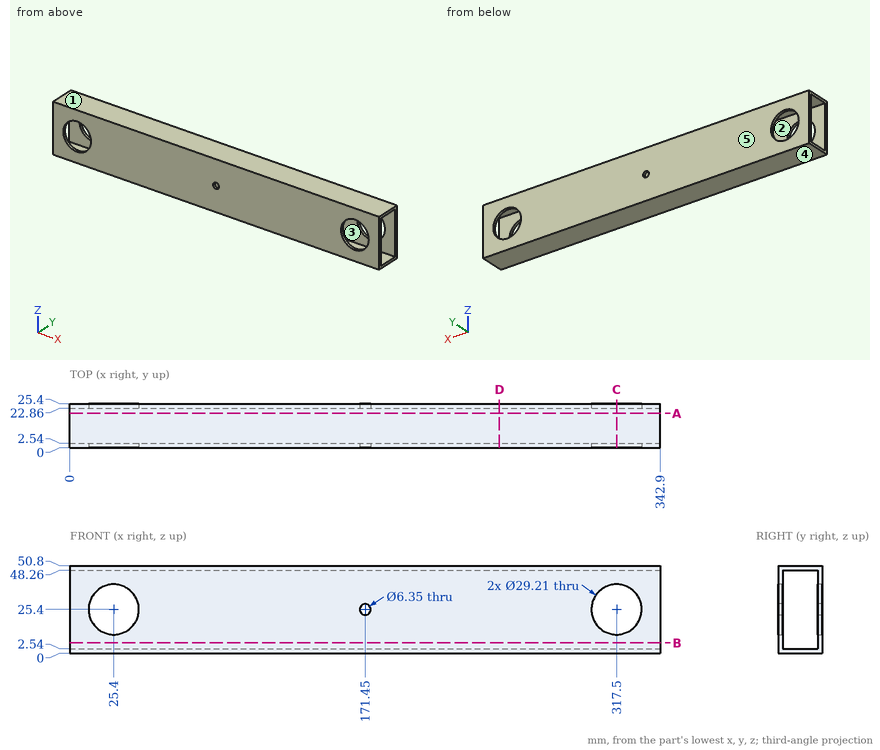
Job drawing, mm, ordinate dimensions from the low corner. One solid piece. A direction names the side the tool comes from. Coordinates: 2 decimals unless noted, no trailing zeros. Loops run counter-clockwise (first coordinate to the right, second up) from the corner with the lowest first, then second, coordinate; pieces in that order, holes last. Notation, with made-up numbers: (-36, -5.75) - (-17, -5.75) arc R19 cw to (-17, 11.25) - close; hole circle Ø3 at (29, 80). An arc over 180 degrees is marked (long way). Answer as a JSON object with one key per item and string values. Group by question number.
(1) Flat gauge pins, fed straight in: pin 1 (1.5 mm diameter, centred on x = 43.5, y = 17, fed in from -Z); pin 2 (10 mm diameter, centred on y = 17.5, z = 20.5, fed in from +X). Where does each tip first touch, or does it go through?
(2) Cut at D-D (x = 249.5). Give the cut face in (y, z).
(3) Two-plate mould, pull along Z, no slides. Class the marked faces 3, 4 and 5: released by +Z, released by -Z, zero draft, split by the parting line, or undercut.
(4) Tool access for the marked faces 1 and 2: list every direction of +Z, -Z, +X, -X, +Y, -Y with a clear straight run to the whole face (end or side of a thin tool).
(5) Cut at C-C (x = 317.5). Give the cut face in (y, z) (3 decimals), then the cut area to 3 significant figures.
(6) Probe line 1 along X through (y, z) = (1.85, 25.4) (3 decimals); line 2 along Z through (x, y) = (82.5, 22.25); line 3 along Y through (x, z) = (36.5, 35). List the from-to ranges inside material, lowest first.
(7) Cut at A-A (y = 20). Give the cut face in (x, z), then the cut area to 3 significant figures.
(8) Cut at B-B (z = 6). Give the cut face in (x, y), then the cut area to 3 significant figures.
Geometry says:
{
 "1": {"pin 1": "stops at z = 0", "pin 2": "passes through"},
 "2": {"outline": "(0, 0) - (25.4, 0) - (25.4, 50.8) - (0, 50.8) - close; hole (2.54, 2.54) - (22.86, 2.54) - (22.86, 48.26) - (2.54, 48.26) - close"},
 "3": {"face 3": "undercut", "face 4": "released by -Z", "face 5": "zero draft"},
 "4": {"face 1": "+Z, +X, -X, +Y, -Y", "face 2": "+X, -X"},
 "5": {"outline": "(0, 0) - (25.4, 0) - (25.4, 10.795) - (22.86, 10.795) - (22.86, 2.54) - (2.54, 2.54) - (2.54, 10.795) - (0, 10.795) - close; (0, 40.005) - (2.54, 40.005) - (2.54, 48.26) - (22.86, 48.26) - (22.86, 40.005) - (25.4, 40.005) - (25.4, 50.8) - (0, 50.8) - close", "area": "213 mm^2"},
 "6": {"line 1": "x = 0 to 10.795, 40.005 to 168.275, 174.625 to 302.895, 332.105 to 342.9", "line 2": "z = 0 to 2.54, 48.26 to 50.8", "line 3": "y = 0 to 2.54, 22.86 to 25.4"},
 "7": {"outline": "(0, 0) - (342.9, 0) - (342.9, 2.54) - (0, 2.54) - close; (0, 48.26) - (342.9, 48.26) - (342.9, 50.8) - (0, 50.8) - close", "area": "1,740 mm^2"},
 "8": {"outline": "(0, 0) - (342.9, 0) - (342.9, 2.54) - (0, 2.54) - close; (0, 22.86) - (342.9, 22.86) - (342.9, 25.4) - (0, 25.4) - close", "area": "1,740 mm^2"}
}
